Here's how the part is built. I have some questions about the finished solid (model axes, mm). Give positions to 0.01 mm unless a question says otherwise; leave off trailing zeros. Write each loop counter-clockwise with the first axis right and the second up, starting at its lowest first coordinate (ties: lowest second). Pieces come first, ordered by that corner, then holes. Notation, with made-up numbers: (-7.5, 15) -> (7.5, 15) arc R36 ccw to (7.5, 54) -> close; hole circle Ø11 at (5, 33.5). An arc over 180 degrees is marked (long way). Use CSV: the item, a comma, the result in double quotes. Start each with the question number.
(1) Suppose I cut it at B-B on x = -15.8. List the corners of the cut face in (y, z) for me (3 decimals), plus the area to 3 significant figures.
(2) Suppose I cut it at C-C on y = 4.45. List the corners of the cut face in (x, z) for me (3 decimals).
(3) Suppose I cut it at A-A on z = -14.55. List the corners of the cut face in (x, y) for me (3 decimals).
(4) If we mould it in two halves opening along X, with no side actions, what happens to faces 1 (the flat face through (-8, 2, -52)), 2 (the cylindrical face through (-9.996, 2.465, -19.872)), 3 (the cylindrical face through (-8.21, 2.46, -46.73)), 4 (the cylindrical face through (-22.58, 2.46, -49.44))? For each: pulls with the +X half, pulls with the -X half, needs draft (parallel to the pull), parting line crosses it, or undercut.
(5) I need wall thicknesses on L1, parallel to Z at x = -15.8, y = 1.8 (3 decimals); L2, parallel to Z at x = -9.5, y = 4.1 (3 decimals); L3, parallel to X at y = 0.5, z = -20.5. Which ranges of each line are inside material? Lowest first, please. Write a range as [from, to].
(6) Suppose I cut it at D-D on x = -8.5. List the corners of the cut face in (y, z) for me, plus the area to 3 significant figures.
Autodesk Inventor part; units mm, degrees
ref_plane "YZ Plane" through (0, 0, 0) normal (1, 0, 0) x (0, 1, 0)
ref_plane "XZ Plane" through (0, 0, 0) normal (0, 1, 0) x (-1, 0, 0)
ref_plane "XY Plane" through (0, 0, 0) normal (0, 0, 1) x (1, 0, 0)
sketch "Sketch1" plane through (0, 0, 0) normal (0, 1, 0) x (-1, 0, 0)
  line L0 (0, 0) -> (25, 0)
  line L1 (25, 0) -> (25, -43.5)
  line L2 (16.5, -52) -> (0, -52)
  line L3 (0, -52) -> (0, 0)
  arc A0 (16.5, -52) -> (25, -43.5) centre (16.5, -43.5) ccw
  circle A1 centre (15.8, -14.55) radius 7.875
  circle A2 centre (8.5, -44.55) radius 2.2
  line L4 (5, 10.2052) -> (5, -72.053) construction
  point P0 (25, -52)
  dimension "d0" = 25
  dimension "d1" = 52
  dimension "d2" = 8.5
  dimension "d3" = 15.75
  dimension "d4" = 4.4
  dimension "d5" = 16.5
  dimension "d6" = 7.45
  dimension "d7" = 20
  dimension "d8" = 9.2
  dimension "d9" = 30
extrude "Extrusion1" add sketch "Sketch1" along normal blind 5
properties part number "corner spacers"
Geometry says:
1,outline,"(0, -52) -> (5, -52) -> (5, -22.425) -> (0, -22.425) -> close; (0, -6.675) -> (5, -6.675) -> (5, 0) -> (0, 0) -> close"
1,area,"181 mm²"
2,outline,"(-25, -43.5) arc R8.5 ccw to (-16.5, -52) -> (0, -52) -> (0, 0) -> (-25, 0) -> close; hole circle Ø15.75 at (-15.8, -14.55); hole circle Ø4.4 at (-8.5, -44.55)"
3,outline,"(-25, 0) -> (-23.675, 0) -> (-23.675, 5) -> (-25, 5) -> close; (-7.925, 0) -> (0, 0) -> (0, 5) -> (-7.925, 5) -> close"
4,face 1,"needs draft"
4,face 2,"undercut"
4,face 3,"undercut"
4,face 4,"pulls with the -X half"
5,L1,"[-52, -22.425], [-6.675, 0]"
5,L2,"[-52, -46.51], [-42.59, -19.275], [-9.825, 0]"
5,L3,"[-25, -20.96], [-10.64, 0]"
6,outline,"(0, -52) -> (5, -52) -> (5, -46.75) -> (0, -46.75) -> close; (0, -42.35) -> (5, -42.35) -> (5, -17.5) -> (0, -17.5) -> close; (0, -11.6) -> (5, -11.6) -> (5, 0) -> (0, 0) -> close"
6,area,"208 mm²"
